```python
from build123d import *

# Parameters (mm, degrees)
SKETCH2_R          = 3.935
SKETCH2_R_2        = 1
CUT_EXTRUDE1_DEPTH = 45


with BuildPart() as part:
    # Sketch1 → Revolve1 (revolve)
    with BuildSketch(Plane.XY, mode=Mode.PRIVATE) as revolve1_sk:
        Polygon((-3, 0), (-3, 20.5), (-10.9, 20.5), (-10.9, 16.5), (-9.855, 15.455), (-9.855, 5.045), (-10.9, 4), (-10.9, 0), align=None)
    revolve(revolve1_sk.sketch.rotate(Axis((0, 0, 0), (0, 1, 0)), 270), axis=Axis((0, 0, 0), (0, 1, 0)))

    # Sketch2 → Cut-Extrude1 (cut)
    with BuildSketch(Plane(origin=(0, 20.5, 0), x_dir=(1, 0, 0), z_dir=(0, 1, 0))):
        with Locations(Location((0, 0, 0), (0, 0, 270))):
            Circle(SKETCH2_R)
        with Locations(Location((-5, 5, 0), (0, 0, 270))):
            Circle(SKETCH2_R_2)
        with Locations(Location((5, 5, 0), (0, 0, 270))):
            Circle(SKETCH2_R_2)
        with Locations(Location((5, -5, 0), (0, 0, 270))):
            Circle(SKETCH2_R_2)
        with Locations(Location((-5, -5, 0), (0, 0, 270))):
            Circle(SKETCH2_R_2)
        with Locations(Location((-7.071067812, 0, 0), (0, 0, 270))):
            Circle(SKETCH2_R_2)
        with Locations(Location((0, 7.071067812, 0), (0, 0, 270))):
            Circle(SKETCH2_R_2)
        with Locations(Location((7.071067812, 0, 0), (0, 0, 270))):
            Circle(SKETCH2_R_2)
        with Locations(Location((0, -7.071067812, 0), (0, 0, 270))):
            Circle(SKETCH2_R_2)
    extrude(amount=-CUT_EXTRUDE1_DEPTH, mode=Mode.SUBTRACT)


solid = part.part
```
Part model, mm, in its own coordinate system. A direction names the side the tool comes from. Round coordinates to 2 decimals unless told otherwise and drop trailing zeros. Answer as CSV lines item,"result". Start each with the question number.
1) Drill centre lines: L1, parallel to X at y = 6.5, z = 0 (3 decimals); L2, parallel to Z at x = -4.75, y = 17.75; L3, parallel to X at y = 12.25, z = -5. Where is each one in solid material? Low to high.
2) Mould opens along X. For faces 3 (the face through (10.64, 18.47, 2.36)), 4 (the face through (0, 20.5, 5)), 5 (the face through (-4, 10, 5)) say: +X half, -X half, draft (parallel to the pull), parting line (faces both ways), or undercut.
3) Band-saw the part on A-A (y = 18.5). Count the separate pieces of the cut face and the enclosed holes in it, then the cut area to 3 significant figures.
4) Which spindle directions (+Z, -Z, +X, -X, +Y, -Y) get a long thin tool onto all of the face, cutting with end or side? Do faces 1 (the face through (-9.77, 10.18, 1.28)), 2 (the face through (6, 10, 5)). Say none if no direction does.
5) Drop flat-ended pins along their axis: pin 1 (5 mm diameter, centred on y = 14, z = -1.5, fed in from -X); pin 2 (1.2 mm diameter, centred on x = 0, z = 7.07, fed in from +Y); pin 3 (1.5 mm diameter, centred on y = 15.5, z = 7.5, fed in from +X); pin 4 (1.5 mm diameter, centred on y = 12.5, z = -4, fed in from +X). Give the stop position or say it passes through.
Worked out:
1,L1,"-9.855 to -8.071, -6.071 to -3.935, 3.935 to 6.071, 8.071 to 9.855"
1,L2,"-9.81 to -5.97, -4.03 to 4.03, 5.97 to 9.81"
1,L3,"-8.49 to -6, -4 to 4, 6 to 8.49"
2,face 3,"parting line"
2,face 4,"draft"
2,face 5,"undercut"
3,separate pieces,"1"
3,enclosed holes,"9"
3,area,"299 mm²"
4,face 1,"none"
4,face 2,"+Y, -Y"
5,pin 1,"x = -10.82"
5,pin 2,"through"
5,pin 3,"x = 7.78"
5,pin 4,"x = 9.3"
